Verification items for the finished model (mm, model axes). A direction names the side the tool comes from. Give positions to 0.01 mm unless a question says otherwise; leave off trailing zeros. Write each loop counter-clockwise with the first axis right and the second up, starting at its lowest first coordinate (ties: lowest second). Pieces come first, ordered by that corner, then holes. Notation, with made-up numbers: M 42.5,43.25 L 59.5,43.25 A23 cw 59.5,75.25 Z; hole C 31.5,87.25 d4. An arc over 180 degrees is marked long. Answer as a JSON object with one key per item and string values.
```python
from build123d import *

# Parameters (mm, degrees)
F0_W     = 24
F0_H     = 54
F1_DEPTH = 40
F2_DEPTH = 5
F3_SIZE  = 2


with BuildPart() as f1:
    # F0 (on Top) → F1 (new body)
    with BuildSketch(Plane.XY):
        Polygon((-15, 29.171573), (-15, 4.171573), (-12.171573, 7), (-12.171573, 0), (-12.171573, -7), (-15, -4.171573), (-15, -29.171573), (15, -29.171573), (15, -3.171573), (17.262742, -5.434315), (17.262742, -0.565685), (17.262742, 0.565685), (17.262742, 5.434315), (15, 3.171573), (15, 29.171573), align=None)
        with Locations((1.500004, 0)):
            Rectangle(F0_W, F0_H, mode=Mode.SUBTRACT)
    extrude(amount=F1_DEPTH)

    # F0 (on Top) → F2 (join)
    with BuildSketch(Plane.XY):
        Polygon((-15, 29.171573), (-15, 4.171573), (-12.171573, 7), (-12.171573, 0), (-12.171573, -7), (-15, -4.171573), (-15, -29.171573), (15, -29.171573), (15, -3.171573), (17.262742, -5.434315), (17.262742, -0.565685), (17.262742, 0.565685), (17.262742, 5.434315), (15, 3.171573), (15, 29.171573), align=None)
        with Locations((1.500004, 0)):
            Rectangle(F0_W, F0_H, mode=Mode.SUBTRACT)
        with Locations((1.500004, 0)):
            Rectangle(F0_W, F0_H)
    extrude(amount=-F2_DEPTH)

    # F3
    f3_edges = [f1.edges().sort_by_distance(p)[0] for p in [
        (0, -29.171573, -5),
        (0, 29.171573, -5),
        (0, -29.171573, 40),
        (0, 29.171573, 40),
    ]]
    chamfer(f3_edges, length=F3_SIZE)


solid = f1.part
```
1) Section check A-A on z = 3.5. Record the boundary of the cut face in (x, y).
Completed:
{"outline": "M -15,-29.17 L 15,-29.17 L 15,-3.17 L 17.26,-5.43 L 17.26,5.43 L 15,3.17 L 15,29.17 L -15,29.17 L -15,4.17 L -12.17,7 L -12.17,-7 L -15,-4.17 Z; hole M -10.5,-27 L 13.5,-27 L 13.5,27 L -10.5,27 Z"}
2) Section check B-B on x = -2. Record the boundary of the cut face in (y, z).
Completed:
{"outline": "M -29.17,-3 L -27.17,-5 L 27.17,-5 L 29.17,-3 L 29.17,38 L 27.17,40 L 27,40 L 27,0 L -27,0 L -27,40 L -27.17,40 L -29.17,38 Z"}
3) Access from +Z, -Z, +X, -X, +Y, -Y to the whole of each face (thin tool, end or side, straight path). Record for faces 5 (the face through (1, 0, -5)), 6 (the face through (-12.172, 0, 18)), 7 (the face through (1, 0, 0)).
Completed:
{"face 5": "-Z, +X, -X, +Y, -Y", "face 6": "+Z, -Z", "face 7": "+Z"}
4) Section check C-C on y = 23. Record the boundary of the cut face in (x, z), and give its area (3 significant figures).
Completed:
{"outline": "M -15,-5 L 15,-5 L 15,40 L 13.5,40 L 13.5,0 L -10.5,0 L -10.5,40 L -15,40 Z", "area": "390 mm2"}
5) Thickness scan on L1, parallel to X at y = 1, z = 19; L2, parallel to X at y = 8, z = 19; L3, parallel to Y at x = 3, z = 0.5. Record the ranges inside material, lowest first.
Completed:
{"L1": "x = -12.17 to -10.5, 13.5 to 17.26", "L2": "x = -15 to -10.5, 13.5 to 15", "L3": "y = -29.17 to -27, 27 to 29.17"}
6) Release check for a two-part mould opening along Y. For faces 1 (the face through (-15, -16, 18)), 2 (the face through (1, 27, 20)), 3 (the face through (0, 29.172, 18)), 4 (the face through (-0.21, -28.16, 39.01)) record: pulls with the +Y half, pulls with the -Y half, needs draft (parallel to the pull), parting line crosses it, or undercut.
Completed:
{"face 1": "needs draft", "face 2": "undercut", "face 3": "pulls with the +Y half", "face 4": "pulls with the -Y half"}
7) Go/stop test with flat-tipped pins: pin 1 (13 mm diameter, centred on y = -15.5, z = 21, fed in from +X); pin 2 (19 mm diameter, centred on x = 0.5, y = 12, fed in from +Z); pin 3 (10 mm diameter, centred on x = 10.5, y = -9, fed in from +Z). Record where each tip stops, or that it passes through.
Completed:
{"pin 1": "stops at x = 15", "pin 2": "stops at z = 0", "pin 3": "stops at z = 40"}
8) Section check D-D on z = -1. Record the boundary of the cut face in (x, y).
Completed:
{"outline": "M -15,-29.17 L 15,-29.17 L 15,-3.17 L 17.26,-5.43 L 17.26,5.43 L 15,3.17 L 15,29.17 L -15,29.17 L -15,4.17 L -12.17,7 L -12.17,-7 L -15,-4.17 Z"}
